The listing builds one solid part. Answer for the finished solid, in the listing's coordinates (mm). Face numbers are marked on the shaded views. A direction names the side the tool comes from. Coordinates: 2 decimals unless noted, no trailing zeros. Order: outer loops, then holes, each group sorted by start corner. A loop starts at its lowest first (then second) coordinate and runs counter-clockwise, first axis right, second up.
from build123d import *

# Parameters (mm, degrees)
SKETCH1_R                = 2
BOSS_EXTRUDE1_DEPTH      = 5
SKETCH2_R                = 1.5
BOSS_EXTRUDE2_DEPTH      = 15
SKETCH3_R                = 1.5
BOSS_EXTRUDE3_DEPTH      = 19.75
CROQUIS1_R               = 1.55
SALIENTE_EXTRUIR1_DEPTH  = 4.5
SALIENTE_EXTRUIR5_REACH  = 73.33
CROQUIS5_W               = 16
CROQUIS5_H               = 35.719654706
SALIENTE_EXTRUIR6_DEPTH  = 24.75
CROQUIS6_W               = 21.702147556
CROQUIS6_H               = 9.928090966
CORTAR_EXTRUIR1_DEPTH    = 13
CORTAR_EXTRUIR2_DEPTH    = 19.75
CROQUIS8_R               = 0.95
CORTAR_EXTRUIR3_DEPTH    = 4.75
SALIENTE_EXTRUIR7_DEPTH  = 3.45
CORTAR_EXTRUIR4_DEPTH    = 3
CORTAR_EXTRUIR5_DEPTH    = 16.5
CROQUIS14_R              = 1.5
SALIENTE_EXTRUIR8_DEPTH  = 1
SIMETR_A5_START          = -1
SIMETR_A5_OUTLINE_R      = 0.95
SIMETR_A5_DEPTH          = 1.3
SALIENTE_EXTRUIR9_START  = -4.5
CROQUIS15_R              = 1.55
SALIENTE_EXTRUIR9_DEPTH  = 4.5
SALIENTE_EXTRUIR10_START = 1
CROQUIS16_R              = 1.55
CROQUIS16_R_2            = 0.95
CROQUIS16_R_3            = 1.5
SALIENTE_EXTRUIR10_DEPTH = 1
CROQUIS17_R              = 2.5
CORTAR_EXTRUIR7_DEPTH    = 2
REDONDEO6_R              = 1
REDONDEO7_R              = 1
REDONDEO8_R              = 1


# Read off the part's stored shape, not the designer's step: Simetría5
with BuildPart() as part:
    # Sketch1 → Boss-Extrude1 (new body)
    with BuildSketch(Plane.XY):
        with BuildLine():
            Line((-8, 0), (-8, 37.32353581))
            Line((-8, 37.32353581), (8, 37.32353581))
            Line((8, 37.32353581), (8, 4.236047978))
            Line((8, 4.236047978), (5.844390358, 4.236047978))
            Line((5.844390358, 4.236047978), (3.979699792, -4.569047459))
            ThreePointArc((3.979699792, -4.569047459), (-3.04298408, -4.99253696), (-8, 0))
        make_face()
        Circle(SKETCH1_R, mode=Mode.SUBTRACT)
    extrude(amount=BOSS_EXTRUDE1_DEPTH)

    # Sketch2 → Boss-Extrude2 (add)
    with BuildSketch(Plane.XY.offset(5)):
        with Locations((0, 30)):
            Circle(SKETCH2_R)
    extrude(amount=BOSS_EXTRUDE2_DEPTH)

    # Sketch3 → Boss-Extrude3 (add)
    with BuildSketch(Plane.XY.offset(5)):
        with BuildLine():
            Line((-2.968624299, 23.290881231), (-2.968624299, 3.203458857))
            Line((-2.968624299, 3.203458857), (5, 3.203458857))
            Line((5, 3.203458857), (5, 0))
            ThreePointArc((5, 0), (3.535533906, -3.535533906), (0, -5))
            Line((0, -5), (-3, -5))
            Line((-3, -5), (-6.244997998, -5))
            ThreePointArc((-6.244997998, -5), (-7.548509256, -2.649529771), (-8, 0))
            Line((-8, 0), (-8, 30))
            Line((-8, 30), (-2.968624299, 23.290881231))
        make_face()
        Circle(SKETCH3_R, mode=Mode.SUBTRACT)
    extrude(amount=BOSS_EXTRUDE3_DEPTH)

    # Croquis1 → Saliente-Extruir1 (add)
    with BuildSketch(Plane.XY.offset(20)):
        with BuildLine():
            Line((8, 30), (8, 60))
            ThreePointArc((8, 60), (0, 68), (-8, 60))
            Line((-8, 60), (-8, 30))
            ThreePointArc((-8, 30), (0, 22), (8, 30))
        make_face()
        with Locations((0, 60)):
            Circle(CROQUIS1_R, mode=Mode.SUBTRACT)
    saliente_extruir1 = extrude(amount=SALIENTE_EXTRUIR1_DEPTH)

    # Saliente-Extruir5: up to this face of the body (flat: up to its plane)
    saliente_extruir5_end = Plane(part.part.faces().sort_by_distance((-0.202248034, 17.4746777, 0))[0])
    # Croquis4 → Saliente-Extruir5 (add, up to the picked face)
    with BuildSketch(Plane(origin=(0, 0, 20), x_dir=(-1, 0, 0), z_dir=(0, 0, -1)), mode=Mode.PRIVATE) as saliente_extruir5_sk1:
        with BuildLine():
            Line((8, 32.729705588), (8, 54.729705588))
            ThreePointArc((8, 54.729705588), (0.622079601, 50.239050865), (-8, 49.729705588))
            Line((-8, 49.729705588), (-8, 32.729705588))
            Line((-8, 32.729705588), (8, 32.729705588))
        make_face()
    saliente_extruir5_tool1 = split(extrude(saliente_extruir5_sk1.sketch, amount=SALIENTE_EXTRUIR5_REACH, mode=Mode.PRIVATE), bisect_by=saliente_extruir5_end, keep=Keep.BOTH, mode=Mode.PRIVATE)
    add(saliente_extruir5_tool1.solids().sort_by(Axis((-0.349387, 41.805362, 20), (0, 0, -1)))[0])

    # Croquis5 → Saliente-Extruir6 (add)
    with BuildSketch(Plane(origin=(0, 0, 0), x_dir=(-1, 0, 0), z_dir=(0, 0, -1))):
        with Locations((0, 22.095875331)):
            Rectangle(CROQUIS5_W, CROQUIS5_H)
    extrude(amount=-SALIENTE_EXTRUIR6_DEPTH)

    # Croquis6 → Cortar-Extruir1 (cut)
    with BuildSketch(Plane(origin=(5, 0, 0), x_dir=(0, 0, -1), z_dir=(1, 0, 0))):
        with Locations((-15.851073778, -1.760586626)):
            Rectangle(CROQUIS6_W, CROQUIS6_H)
    extrude(amount=-CORTAR_EXTRUIR1_DEPTH, mode=Mode.SUBTRACT)

    # Croquis7 → Cortar-Extruir2 (cut)
    with BuildSketch(Plane.XY.offset(24.75)):
        with BuildLine():
            Line((-8, 3.203458857), (8, 3.203458857))
            Line((8, 3.203458857), (8, 3.520097758))
            ThreePointArc((8, 3.520097758), (-0.079264703, 7.367082887), (-8, 3.203458857))
        make_face()
    extrude(amount=-CORTAR_EXTRUIR2_DEPTH, mode=Mode.SUBTRACT)

    # Croquis8 → Cortar-Extruir3 (cut)
    with BuildSketch(Plane.XY.offset(24.75)):
        with Locations((3.5, 48)):
            Circle(CROQUIS8_R)
        with Locations((-3.5, 48)):
            Circle(CROQUIS8_R)
    cortar_extruir3 = extrude(amount=-CORTAR_EXTRUIR3_DEPTH, mode=Mode.SUBTRACT)

    # Croquis9 → Saliente-Extruir7 (add, symmetric)
    with BuildSketch(Plane.XY.offset(24.75)):
        with BuildLine():
            Line((-8, 40.520097758), (-8, 3.203458857))
            ThreePointArc((-8, 3.203458857), (-0.665608426, 7.324319495), (7.159822628, 4.236047978))
            Line((7.159822628, 4.236047978), (8, 4.236047978))
            Line((8, 4.236047978), (8, 49.729705588))
            ThreePointArc((8, 49.729705588), (-0.622079601, 50.239050865), (-8, 54.729705588))
            Line((-8, 54.729705588), (-8, 40.520097758))
        make_face()
    extrude(amount=SALIENTE_EXTRUIR7_DEPTH, both=True)

    # Simetría1: part across plane


with BuildPart() as part_1:
    add(part.part)
    add(part.part.mirror(Plane(origin=(4.712433071, 67.309491417, 28.2), x_dir=(1, 0, 0), z_dir=(0, 0, -1))))

    # Croquis10 → Cortar-Extruir4 (cut)
    with BuildSketch(Plane(origin=(0, 0, 31.9), x_dir=(-1, 0, 0), z_dir=(0, 0, -1))):
        Polygon((2.51627812, 61.936924819), (-0.419287038, 63.147623185), (-2.935565159, 61.210698366), (-2.51627812, 58.063075181), (0.419287038, 56.852376815), (2.935565159, 58.789301634), align=None)
    extrude(amount=-CORTAR_EXTRUIR4_DEPTH, mode=Mode.SUBTRACT)

    # Simetría3: Saliente-Extruir1, Cortar-Extruir3 across plane
    add(saliente_extruir1.mirror(Plane.XY.offset(38.7)))
    add(cortar_extruir3.mirror(Plane.XY.offset(38.7)), mode=Mode.SUBTRACT)

    # Croquis12 → Cortar-Extruir5 (cut, symmetric)
    with BuildSketch(Plane.XY.offset(36.4)):
        with BuildLine():
            Line((-8, 54.729705588), (-10.312115974, 60.381035393))
            Line((-10.312115974, 60.381035393), (-8.568993542, 74.199141583))
            Line((-8.568993542, 74.199141583), (17.131520351, 70.957080647))
            Line((17.131520351, 70.957080647), (14.495741362, 50.062694062))
            Line((14.495741362, 50.062694062), (8, 49.729705588))
            ThreePointArc((8, 49.729705588), (-0.622079601, 50.239050865), (-8, 54.729705588))
        make_face()
    extrude(amount=CORTAR_EXTRUIR5_DEPTH, both=True, mode=Mode.SUBTRACT)

    # Croquis14 → Saliente-Extruir8 (add)
    with BuildSketch(Plane(origin=(0, 0, 0), x_dir=(-1, 0, 0), z_dir=(0, 0, -1))):
        with BuildLine():
            Line((-8, 49.729705588), (-8, 4.236047978))
            Line((-8, 4.236047978), (-5.844390358, 4.236047978))
            Line((-5.844390358, 4.236047978), (-3.979699792, -4.569047459))
            ThreePointArc((-3.979699792, -4.569047459), (3.04298408, -4.99253696), (8, 0))
            Line((8, 0), (8, 54.729705588))
            ThreePointArc((8, 54.729705588), (0.622079601, 50.239050865), (-8, 49.729705588))
        make_face()
        Circle(CROQUIS14_R, mode=Mode.SUBTRACT)
    extrude(amount=SALIENTE_EXTRUIR8_DEPTH)

    # Simetría5 outline → Simetría5 (cut)
    with BuildSketch(Plane.XY.offset(SIMETR_A5_START)):
        with Locations((-3.5, 48)):
            Circle(SIMETR_A5_OUTLINE_R)
        with Locations((3.5, 48)):
            Circle(SIMETR_A5_OUTLINE_R)
    extrude(amount=SIMETR_A5_DEPTH, mode=Mode.SUBTRACT)

    # Croquis15 → Saliente-Extruir9 (add)
    with BuildSketch(Plane(origin=(0, 0, -1), x_dir=(-1, 0, 0), z_dir=(0, 0, -1)).offset(SALIENTE_EXTRUIR9_START)):
        with BuildLine():
            Line((-8, 49.729705588), (-8, 60))
            ThreePointArc((-8, 60), (0, 68), (8, 60))
            Line((8, 60), (8, 54.729705588))
            ThreePointArc((8, 54.729705588), (0.622079601, 50.239050865), (-8, 49.729705588))
        make_face()
        with Locations(Location((0, 60, 0), (0, 0, 180))):
            Circle(CROQUIS15_R, mode=Mode.SUBTRACT)
    extrude(amount=SALIENTE_EXTRUIR9_DEPTH)

    # Croquis16 → Saliente-Extruir10 (add)
    with BuildSketch(Plane.XY.offset(56.4).offset(SALIENTE_EXTRUIR10_START)):
        with BuildLine():
            Line((-8, 0), (-8, 60))
            ThreePointArc((-8, 60), (0, 68), (8, 60))
            Line((8, 60), (8, 4.236047978))
            Line((8, 4.236047978), (5.844390358, 4.236047978))
            Line((5.844390358, 4.236047978), (3.979699792, -4.569047459))
            ThreePointArc((3.979699792, -4.569047459), (-3.04298408, -4.99253696), (-8, 0))
        make_face()
        with Locations((0, 60)):
            Circle(CROQUIS16_R, mode=Mode.SUBTRACT)
        with Locations(Location((3.5, 48, 0), (0, 0, 180))):
            Circle(CROQUIS16_R_2, mode=Mode.SUBTRACT)
        with Locations(Location((-3.5, 48, 0), (0, 0, 180))):
            Circle(CROQUIS16_R_2, mode=Mode.SUBTRACT)
        with Locations(Location((0, 0, 0), (0, 0, 180))):
            Circle(CROQUIS16_R_3, mode=Mode.SUBTRACT)
    extrude(amount=-SALIENTE_EXTRUIR10_DEPTH)

    # Croquis17 → Cortar-Extruir7 (cut)
    with BuildSketch(Plane(origin=(0, 0, -1), x_dir=(-1, 0, 0), z_dir=(0, 0, -1))):
        with Locations((0, 60)):
            Circle(CROQUIS17_R)
    cortar_extruir7 = extrude(amount=-CORTAR_EXTRUIR7_DEPTH, mode=Mode.SUBTRACT)

    # Simetría6: Cortar-Extruir7 across plane
    add(cortar_extruir7.mirror(Plane.XY.offset(28.3)), mode=Mode.SUBTRACT)

    # Redondeo6
    # the kernel refuses this fillet: 1 mm, written as the material it takes off along each edge
    with BuildSketch(Plane(origin=(-8, 60, -1), x_dir=(0, 0, 1), z_dir=(0, -1, 0)), Plane(origin=(-8, -2.5, 57.4), x_dir=(0, 0, -1), z_dir=(0, 1, 0))) as redondeo6_piece_1:
        with BuildLine():
            CenterArc((REDONDEO6_R, -REDONDEO6_R), REDONDEO6_R, 90, 90)
            Line((0, -REDONDEO6_R), (0, 0))
            Line((0, 0), (REDONDEO6_R, 0))
        make_face()
    extrude(amount=62.5, mode=Mode.SUBTRACT)
    with BuildSketch(Plane(origin=(0, 60, -1), x_dir=(1, 0, 0), z_dir=(0, -1, 0))) as redondeo6_piece_2:
        with BuildLine():
            CenterArc((8 - REDONDEO6_R, REDONDEO6_R), REDONDEO6_R, 270, 90)
            Line((8 - REDONDEO6_R, 0), (8, 0))
            Line((8, 0), (8, REDONDEO6_R))
        make_face()
    revolve(axis=Axis((0, 60, -1), (0, 0, 1)), revolution_arc=180, mode=Mode.SUBTRACT)
    with BuildSketch(Plane(origin=(8, 60, -1), x_dir=(-1, 0, 0), z_dir=(0, -1, 0))) as redondeo6_piece_3:
        with BuildLine():
            CenterArc((REDONDEO6_R, -REDONDEO6_R), REDONDEO6_R, 90, 90)
            Line((0, -REDONDEO6_R), (0, 0))
            Line((0, 0), (REDONDEO6_R, 0))
        make_face()
    extrude(amount=58.263952022, mode=Mode.SUBTRACT)
    with BuildSketch(Plane(origin=(8, 4.236047978, 59.9), x_dir=(0, 1, 0), z_dir=(0, 0, -1))) as redondeo6_piece_4:
        with BuildLine():
            CenterArc((REDONDEO6_R, -REDONDEO6_R), REDONDEO6_R, 90, 90)
            Line((0, -REDONDEO6_R), (0, 0))
            Line((0, 0), (REDONDEO6_R, 0))
        make_face()
    extrude(amount=63.4, mode=Mode.SUBTRACT)
    with BuildSketch(Plane(origin=(8, 60, 57.4), x_dir=(-1, 0, 0), z_dir=(0, -1, 0))) as redondeo6_piece_5:
        with BuildLine():
            CenterArc((REDONDEO6_R, REDONDEO6_R), REDONDEO6_R, 180, 90)
            Line((0, REDONDEO6_R), (0, 0))
            Line((0, 0), (REDONDEO6_R, 0))
        make_face()
    extrude(amount=58.263952022, mode=Mode.SUBTRACT)
    with BuildSketch(Plane(origin=(0, 60, 57.4), x_dir=(1, 0, 0), z_dir=(0, -1, 0))) as redondeo6_piece_6:
        with BuildLine():
            CenterArc((8 - REDONDEO6_R, -REDONDEO6_R), REDONDEO6_R, 0, 90)
            Line((8, -REDONDEO6_R), (8, 0))
            Line((8, 0), (8 - REDONDEO6_R, 0))
        make_face()
    revolve(axis=Axis((0, 60, 57.4), (0, 0, 1)), revolution_arc=180, mode=Mode.SUBTRACT)

    # Redondeo7
    redondeo7_edges = [part_1.edges().sort_by_distance(p)[0] for p in [
        (8, 49.729705588, 28.2),
    ]]
    fillet(redondeo7_edges, radius=REDONDEO7_R)

    # Redondeo8
    redondeo8_edges = [part_1.edges().sort_by_distance(p)[0] for p in [
        (-8, 54.729705588, 28.2),
    ]]
    fillet(redondeo8_edges, radius=REDONDEO8_R)


solid = part_1.part
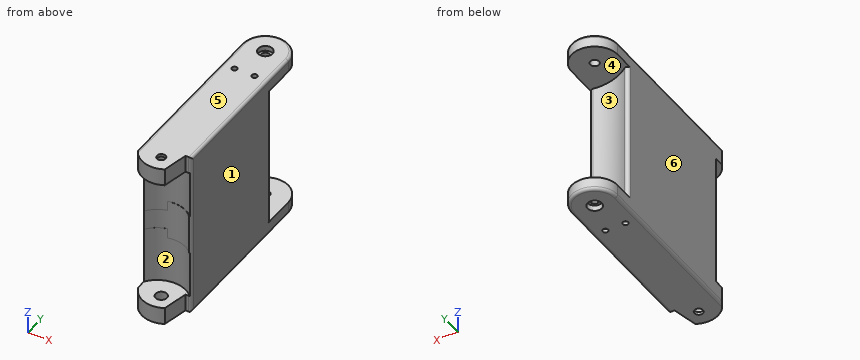
1) Consider L1, parallel to Z at x = -0.5, y = 51.5; L2, parallel to Y at x = 0, z = 57.2; L3, parallel to Y at x = -5, z = 32. Determine where each line is inside the solid, lowest interval first.
2) Determine the mould class of the marked faces 4, 5 and 6 for opening direction Z: released by +Z, released by -Z, zero draft, split by the parting line, or undercut.
3) Each of these flat-tipped pins is pushed along its axis until it touches: P1, Ø1.1, axis at x = 3.5, y = 48, coming from the +Z side; P2, Ø0.6, axis at x = 3.5, y = 48.5, coming from the -Z side; P3, Ø2.5, axis at x = 3.5, y = 48, coming from the +Z side; P4, Ø3, axis at x = 0, y = 60, coming from the -Z side. Where does it stop, or does it pass through?
4) Section D-D (z = 38) is taken. Give the vertices of the cut face in (x, y), then the cut area to 3 significant figures.
5) A tool of negligible diameter and unlimited length cuts with its end or side. For the marked faces 1, 2 and 3, from which of +Z, -Z, +X, -X, +Y, -Y can it reach the whole face along a straight path? Write none if from no direction.
6) Section B-B (x = 0) is taken. Give the number of separate pieces and of enclosed holes in the cut face, then the cut area to 3 significant figures.
7) Section A-A (z = 29) is taken. Give the vertices of the cut face in (x, y), then the cut area to 3 significant figures.
Filled sheet:
1. L1: z = -1 to 3.5, 52.9 to 57.4
1. L2: y = -5.55 to -1.5, 1.5 to 57.5, 62.5 to 67.6
1. L3: y = 5.96 to 52.29
2. face 4: undercut
2. face 5: released by +Z
2. face 6: zero draft
3. P1: stops at z = 52.65
3. P2: stops at z = 0.3
3. P3: stops at z = 57.4
3. P4: passes through
4. outline: (-8, 3.2) arc R9.99 cw to (7.33, 4.29) arc R1 ccw to (8, 5.24) - (8, 48.56) arc R1 ccw to (6.88, 49.56) arc R17.88 cw to (-6.38, 53.28) arc R1 ccw to (-8, 52.5) - close
4. area: 712 mm2
5. face 1: +Z, -Z, +X, +Y, -Y
5. face 2: -Y
5. face 3: +Y
6. separate pieces: 5
6. enclosed holes: 0
6. area: 2,730 mm2
7. outline: (-8, 3.2) arc R9.79 cw to (7.15, 4.25) arc R1 ccw to (8, 5.24) - (8, 48.56) arc R1 ccw to (6.88, 49.56) arc R17.88 cw to (-6.38, 53.28) arc R1 ccw to (-8, 52.5) - close
7. area: 712 mm2
